```python
from build123d import *

# Parameters (mm, degrees)
F1_DEPTH      = 6.35
F0_W          = 12.7
F0_H          = 76.2
F2_DEPTH      = 23.114
F2_DEPTH_BACK = 7.62
F3_W          = 13.847873
F3_H          = 81.732566
F4_DEPTH      = 70.104
F4_DEPTH_BACK = 9.652
F5_W          = 60.452
F5_H          = 13.946542
F6_DEPTH      = 11.43


with BuildPart() as f1:
    # F0 (on Front) → F1 (new body, symmetric)
    with BuildSketch(Plane.XZ):
        Polygon((38.65377, -59.13078), (51.35377, -59.13078), (51.35377, -21.038081), (51.35377, -14.115668), (38.65377, -14.115668), (38.65377, 62.084332), (51.35377, 62.084332), (51.35377, 68.237185), (51.35377, 99.61922), (-34.49823, 99.61922), (-34.49823, 69.908112), (-34.49823, 62.084332), (-21.79823, 62.084332), (-21.79823, -14.115668), (-34.49823, -14.115668), (-34.49823, -20.321971), (-34.49823, -59.13078), (-30.726077, -59.13078), (-21.79823, -59.13078), (-21.79823, -45.147181), (38.65377, -45.147181), align=None)
        with BuildLine():
            Line((-34.49823, 99.61922), (51.35377, 99.61922))
            ThreePointArc((51.35377, 99.61922), (8.42777, 138.122584), (-34.49823, 99.61922))
        make_face()
    extrude(amount=F1_DEPTH, both=True)

    # F0 (on Front) → F2 (join, two sides)
    with BuildSketch(Plane.XZ) as f2_sk:
        with Locations((-28.14823, 23.984332)):
            Rectangle(F0_W, F0_H)
        with Locations((45.00377, 23.984332)):
            Rectangle(F0_W, F0_H)
        Polygon((35.63362, -59.13078), (38.65377, -59.13078), (38.65377, -45.147181), (-21.79823, -45.147181), (-21.79823, -59.13078), align=None)
    extrude(amount=F2_DEPTH)
    extrude(f2_sk.sketch, amount=-F2_DEPTH_BACK)

    # F3 (on face) → F4 (cut, two sides)
    with BuildSketch(Plane.YZ.offset(-21.79823)) as f4_sk:
        with Locations((-13.503438, 23.114669)):
            Rectangle(F3_W, F3_H)
    extrude(amount=F4_DEPTH, mode=Mode.SUBTRACT)
    extrude(f4_sk.sketch, amount=-F4_DEPTH_BACK, mode=Mode.SUBTRACT)

    # F5 (on face) → F6 (cut)
    with BuildSketch(Plane.XY.offset(-45.147181)):
        with Locations((8.42777, -13.323271)):
            Rectangle(F5_W, F5_H)
    extrude(amount=-F6_DEPTH, mode=Mode.SUBTRACT)


solid = f1.part
```
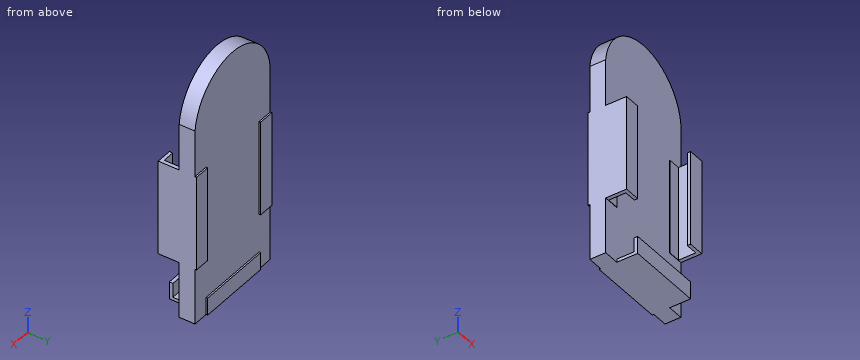
CAD build for the part. Positions are in the model's coordinates, mm. Round coordinates to 2 decimals unless told otherwise and drop trailing zeros. Order: outer loops, then holes, each group sorted by start corner. A loop starts at its lowest first (then second) coordinate and runs counter-clockwise, first axis right, second up.
Q1. Slice it at C-C (z = 46.5). Write the cut outline in (x, y).
Q2. Slice it at B-B (x = -27.5). Write the cut outline in (y, z).
Q3. Slice it at A-A (y = -12). Write the cut outline in (x, z), and give its area (3 significant figures).
Q4. Drop flat-ended pins along their axis: pin 1 (4 mm diameter, centred on x = -30.5, y = -15, fed in from -Z); pin 2 (10 mm diameter, centred on x = 19, z = -24, fed in from -Y); pin 3 (2 mm diameter, centred on x = -1, y = -8, fed in from +Z). Give the stop position or say it passes through.
Q5. Wall check: L1, parallel to Y at x = 40, z = -2.5; L2, parallel to X at y = -12.5, z = -14; L3, parallel to Z at x = 36, y = -21. Give the ranges that are in metal, low to high.
Q6. Slice it at D-D (y = -3). Write the cut outline in (x, z), and give its area (3 significant figures).
Results below:
1. outline: (-34.5, -23.11) - (-21.8, -23.11) - (-21.8, -20.43) - (-31.45, -20.43) - (-31.45, -6.58) - (-21.8, -6.58) - (-21.8, -6.35) - (38.65, -6.35) - (38.65, -6.58) - (48.31, -6.58) - (48.31, -20.43) - (38.65, -20.43) - (38.65, -23.11) - (51.35, -23.11) - (51.35, 7.62) - (38.65, 7.62) - (38.65, 6.35) - (-21.8, 6.35) - (-21.8, 7.62) - (-34.5, 7.62) - close
2. outline: (-23.11, -14.12) - (-20.43, -14.12) - (-20.43, 62.08) - (-23.11, 62.08) - close; (-6.58, -14.12) - (-6.35, -14.12) - (-6.35, -59.13) - (6.35, -59.13) - (6.35, -14.12) - (7.62, -14.12) - (7.62, 62.08) - (6.35, 62.08) - (6.35, 118.89) - (-6.35, 118.89) - (-6.35, 62.08) - (-6.58, 62.08) - close
3. outline: (-34.5, -14.12) - (-31.45, -14.12) - (-31.45, 62.08) - (-34.5, 62.08) - close; (-21.8, -59.13) - (38.65, -59.13) - (38.65, -56.58) - (-21.8, -56.58) - close; (48.31, -14.12) - (51.35, -14.12) - (51.35, 62.08) - (48.31, 62.08) - close
3. area: 619 mm2
4. pin 1: stops at z = -14.12
4. pin 2: stops at y = -6.35
4. pin 3: stops at z = -56.58
5. L1: y = -23.11 to -20.43, -6.58 to 7.62
5. L2: x = -34.5 to -31.45, 48.31 to 51.35
5. L3: z = -59.13 to -45.15
6. outline: (-34.5, -59.13) - (51.35, -59.13) - (51.35, 99.62) arc R43.18 ccw to (-34.5, 99.62) - close
6. area: 16,200 mm2
